Autodesk Fusion 360 part; units mm, degrees
sketch "Sketch1" plane through (0, 0, 0) normal (0, 0, 1) x (1, 0, 0)
  line L0 (0, 0) -> (171, 0)
  line L1 (171, 0) -> (171, 80)
  line L2 (171, 80) -> (0, 80)
  line L3 (0, 80) -> (0, 0)
  dimension "d1" = 80
  dimension "d2" = 171
extrude "Extrude1" add sketch "Sketch1" along normal blind 7
sketch "Sketch2" plane through (0, 0, 7) normal (0, 0, 1) x (-1, 0, 0)
  line L0 (0, -80) -> (0, 0)
  line L1 (0, 0) -> (-171, 0)
  line L2 (-171, 0) -> (-171, -80)
  line L3 (-171, -80) -> (0, -80)
  line L4 (0, 0) -> (-15, 0)
  line L5 (-15, 0) -> (-15, -15)
  line L6 (-15, -15) -> (0, -15)
  line L7 (0, -15) -> (0, 0)
  line L8 (-85.5, 0) -> (-85.5, -80)
  line L9 (-156, 0) -> (-156, -15)
  line L10 (-156, -15) -> (-171, -15)
  line L11 (-171, -15) -> (-171, 0)
  line L12 (-171, 0) -> (-156, 0)
  line L13 (0, -40) -> (-171, -40)
  line L14 (-15, -65) -> (0, -65)
  line L15 (0, -65) -> (0, -80)
  line L16 (0, -80) -> (-15, -80)
  line L17 (-15, -80) -> (-15, -65)
  line L18 (-156, -80) -> (-156, -65)
  line L19 (-156, -65) -> (-171, -65)
  line L20 (-171, -65) -> (-171, -80)
  line L21 (-171, -80) -> (-156, -80)
  dimension "d5" = 15
  dimension "d6" = 15
extrude "Extrude2" add sketch "Sketch2" along normal blind 23 contours L0 L3 L14 L15 L16 L17 | L0 L1 L4 L5 L6 L7 | L2 L3 L18 L19 L20 L21 | L1 L2 L9 L10 L11 L12
sketch "Sketch3" plane through (0, 0, 0) normal (0, 0, -1) x (1, 0, 0)
  line L0 (0, 0) -> (0, -80)
  line L1 (0, -80) -> (171, -80)
  line L2 (171, -80) -> (171, 0)
  line L3 (171, 0) -> (0, 0)
  line L4 (166.5, -4.5) -> (4.5, -4.5)
  line L5 (4.5, -4.5) -> (4.5, -75.5)
  line L6 (4.5, -75.5) -> (166.5, -75.5)
  line L7 (166.5, -75.5) -> (166.5, -4.5)
  dimension "d9" = 4.5
  dimension "d10" = 4.5
  dimension "d11" = 4.5
  dimension "d12" = 4.5
extrude "Extrude3" add sketch "Sketch3" along normal blind 3
Read the model definition and answer for the solid it produces. Units are mm, in the model's axes. A direction names the side the tool comes from. Coordinates: 2 decimals unless noted, no trailing zeros. Order: outer loops, then holes, each group sorted by start corner. A loop starts at its lowest first (then second) coordinate and runs counter-clockwise, first axis right, second up. Notation, with made-up numbers: (33.5, 0) -> (62.5, 0) arc R33 ccw to (62.5, 31) -> close; hole circle Ø3 at (-8, -28). An arc over 180 degrees is marked (long way). Answer as a JSON object with one key per item and string values.
1) A tool of negligible diameter and unlimited length cuts with its end or side. For faces 1 (the face through (87, 4.5, -1)), 2 (the face through (8, 65, 18)), 3 (the face through (156, 73, 18)), 4 (the face through (85, 4, -3)), from which of +Z, -Z, +X, -X, +Y, -Y can it reach the whole face along a straight path? Write none if from no direction.
Model answer:
{"face 1": "-Z", "face 2": "+Z, +X, -X", "face 3": "+Z, +Y, -Y", "face 4": "-Z, +X, -X, +Y, -Y"}
2) Consider line 1 along X through (y, z) = (74.5, 10); line 2 along X through (y, z) = (61, -0.5); line 3 along Z through (x, y) = (42.5, 22). Determine where each line is inside the solid, lowest interval first. Write a range as from..to.
Model answer:
{"line 1": "x = 0..15, 156..171", "line 2": "x = 0..4.5, 166.5..171", "line 3": "z = 0..7"}
3) This flat-tipped pin is pushed along its axis until it touches: pin 1 (4 mm diameter, centred on x = 36, y = 66.5, fed in from +Z). Where does it stop, or does it pass through?
Model answer:
{"pin 1": "stops at z = 7"}
4) A cutting plane is placed at A-A, the plane z = 19. Determine the outline of the cut face in (x, y), plus the area to 3 significant figures.
Model answer:
{"outline": "(0, 0) -> (15, 0) -> (15, 15) -> (0, 15) -> close; (0, 65) -> (15, 65) -> (15, 80) -> (0, 80) -> close; (156, 0) -> (171, 0) -> (171, 15) -> (156, 15) -> close; (156, 65) -> (171, 65) -> (171, 80) -> (156, 80) -> close", "area": "900 mm²"}
5) A cutting plane is placed at B-B, the plane x = 48. Determine the outline of the cut face in (y, z), plus the area to 3 significant figures.
Model answer:
{"outline": "(0, -3) -> (4.5, -3) -> (4.5, 0) -> (75.5, 0) -> (75.5, -3) -> (80, -3) -> (80, 7) -> (0, 7) -> close", "area": "587 mm²"}
6) A cutting plane is placed at D-D, the plane y = 72.5. Determine the outline of the cut face in (x, z), plus the area to 3 significant figures.
Model answer:
{"outline": "(0, -3) -> (4.5, -3) -> (4.5, 0) -> (166.5, 0) -> (166.5, -3) -> (171, -3) -> (171, 30) -> (156, 30) -> (156, 7) -> (15, 7) -> (15, 30) -> (0, 30) -> close", "area": "1,910 mm²"}
7) The mould has two halves that part along X. Classify faces 5 (the face through (0, 39, 6)), 6 (the face through (156, 7, 18)), 7 (the face through (164, 72, 30)): released by +X, released by -X, zero draft, split by the parting line, or undercut.
Model answer:
{"face 5": "released by -X", "face 6": "undercut", "face 7": "zero draft"}
8) A cutting plane is placed at C-C, the plane y = 36. Determine the outline of the cut face in (x, z), plus the area to 3 significant figures.
Model answer:
{"outline": "(0, -3) -> (4.5, -3) -> (4.5, 0) -> (166.5, 0) -> (166.5, -3) -> (171, -3) -> (171, 7) -> (0, 7) -> close", "area": "1,220 mm²"}
